Verification items for the finished model (mm, model axes). A direction names the side the tool comes from. Round coordinates to 2 decimals unless told otherwise and drop trailing zeros. Order: outer loops, then holes, each group sorted by start corner. A loop starts at its lowest first (then second) coordinate and runs counter-clockwise, first axis right, second up. Notation, with made-up numbers: M -23.5,80.25 L -12.5,80.25 A31 cw -12.5,116.25 Z; hole C 84.5,74.5 d4. An arc over 180 degrees is marked long. Answer as a JSON object with one key per item and string values. Group by question number.
Autodesk Inventor part; units mm, degrees
ref_plane "YZ Plane" through (0, 0, 0) normal (1, 0, 0) x (0, 1, 0)
ref_plane "XZ Plane" through (0, 0, 0) normal (0, 1, 0) x (-1, 0, 0)
ref_plane "XY Plane" through (0, 0, 0) normal (0, 0, 1) x (1, 0, 0)
sketch "Sketch1" plane through (0, 0, 0) normal (0, 1, 0) x (-1, 0, 0)
  circle A0 centre (0, 0) radius 8
  dimension "d0" = 16
extrude "Extrusion1" add sketch "Sketch1" along normal blind 7.4
sketch "Sketch2" plane through (0, 7.4, 0) normal (0, 1, 0) x (1, 0, 0)
  circle A0 centre (0, 0) radius 6
  dimension "d3" = 12
extrude "Extrusion2" add sketch "Sketch2" along normal blind 7.1
sketch "Sketch3" plane through (0, 14.5, 0) normal (0, 1, 0) x (1, 0, 0)
  circle A0 centre (0, 0) radius 8
extrude "Extrusion3" add sketch "Sketch3" along normal blind 1
sketch "Sketch4" plane through (0, 15.5, 0) normal (0, 1, 0) x (1, 0, 0)
  circle A0 centre (0, 0) radius 2.5
  dimension "d8" = 5
extrude "Extrusion4" cut sketch "Sketch4" against normal through all
properties part number "GT2 20T"
Q1. Release check for a two-part mould opening along Y. For faces 1 (the face through (-1.73, 14.99, -7.81)), 2 (the face through (-2, 15.5, 2)), 3 (the face through (2, 0, -2)), 4 (the face through (-2, 14.5, -6)) record: released by +Y, released by -Y, zero draft, split by the parting line, or undercut.
Q2. Thickness scan on line 1 (Z direction, x = 0, y = 5.5); line 2 (Y direction, x = -4, z = -6.75); line 3 (X direction, y = 8.75, z = 0). Record the ranges inside material, lowest first. Write a range as from..to.
Q3. Cross-section at A-A, the plane x = 0. Record the cut outline in (y, z).
Q4. Cross-section at D-D, the plane x = -7. Record the cut outline in (y, z).
Q5. Tool access check on faces 5 (the face through (-6, 11, 0)), 6 (the face through (-0.54, 7.86, 2.44)). Record the directions out of +Z, -Z, +X, -X, +Y, -Y that give a thin tool (end or side, any length) a straight path to the whole face; none if there is none.
Q6. Gauge pin test, flat ends, axial feed: pin 1 Ø4 at (x, y) = (-3.5, 12) entering from +Z; pin 2 Ø2 at (x, y) = (-0.5, 11) entering from +Z; pin 3 Ø6 at (x, y) = (3, 7.5) entering from -Z; pin 4 Ø4 at (x, z) = (0, 0) entering from -Y. Record the tip position at first contact, or that the pin passes through.
Q7. Cross-section at C-C, the plane y = 10.5. Record the cut outline in (x, z).
Q8. Cross-section at B-B, the plane z = 0. Record the cut outline in (x, y), then the cut area to 3 significant figures.
Conclusion:
{
 "1": {"face 1": "zero draft", "face 2": "released by +Y", "face 3": "released by -Y", "face 4": "undercut"},
 "2": {"line 1": "-8..-2.5, 2.5..8", "line 2": "0..7.4, 14.5..15.5", "line 3": "-6..-2.5, 2.5..6"},
 "3": {"outline": "M 0,-8 L 7.4,-8 L 7.4,-6 L 14.5,-6 L 14.5,-8 L 15.5,-8 L 15.5,-2.5 L 0,-2.5 Z; M 0,2.5 L 15.5,2.5 L 15.5,8 L 14.5,8 L 14.5,6 L 7.4,6 L 7.4,8 L 0,8 Z"},
 "4": {"outline": "M 0,-3.87 L 7.4,-3.87 L 7.4,3.87 L 0,3.87 Z; M 14.5,-3.87 L 15.5,-3.87 L 15.5,3.87 L 14.5,3.87 Z"},
 "5": {"face 5": "none", "face 6": "+Y, -Y"},
 "6": {"pin 1": "z = 5.81", "pin 2": "z = 6", "pin 3": "z = -8", "pin 4": "through"},
 "7": {"outline": "C 0,0 d12; hole C 0,0 d5"},
 "8": {"outline": "M -8,0 L -2.5,0 L -2.5,15.5 L -8,15.5 L -8,14.5 L -6,14.5 L -6,7.4 L -8,7.4 Z; M 2.5,0 L 8,0 L 8,7.4 L 6,7.4 L 6,14.5 L 8,14.5 L 8,15.5 L 2.5,15.5 Z", "area": "142 mm2"}
}
